Job drawing, mm, ordinate dimensions from the low corner. One solid piece. A direction names the side the tool comes from. Coordinates: 2 decimals unless noted, no trailing zeros. Write each loop counter-clockwise with the first axis right and the second up, starting at its lowest first coordinate (ties: lowest second). Pieces come first, ordered by that corner, then holes. Notation, with made-up numbers: (83, -38) - (124, -38) arc R17 cw to (124, -12) - close; hole circle Ø3 at (-20, 26.5). An arc over 180 degrees is marked (long way). Put each result on its own line as item: value. Start each with the question number.
1. Drop flat-ended pins along their axis: P1, Ø12, axis at y = 4, z = 52, coming from the +X side; P2, Ø9, axis at x = 21, y = 20.5, coming from the +Z side; P3, Ø3, axis at y = 8.5, z = 58.5, coming from the +X side. Give the stop position or say it passes through.
2. Saw through at B-B, the plane z = 33. Write the cut outline in (x, y), plus the area to 3 significant figures.
3. Saw through at C-C, the plane x = 54.5. Write the cut outline in (y, z), plus the area to 3 significant figures.
4. Saw through at A-A, the plane y = 9. Write the cut outline in (x, z).
5. Saw through at D-D, the plane z = 63. Write the cut outline in (x, y), plus the area to 3 significant figures.
6. Which spindle directions (+Z, -Z, +X, -X, +Y, -Y) get a long thin tool onto all of the face, cutting with end or side? Do the marked faces 1 and 2. Say none if no direction does.
7. Drill centre lines: L1, parallel to Z at x = 29, y = 10.25; L2, parallel to X at y = 16.5, z = 66; L3, parallel to X at y = 15.5, z = 35. Where is each one in solid material? Low to high. Write a range as from..to.
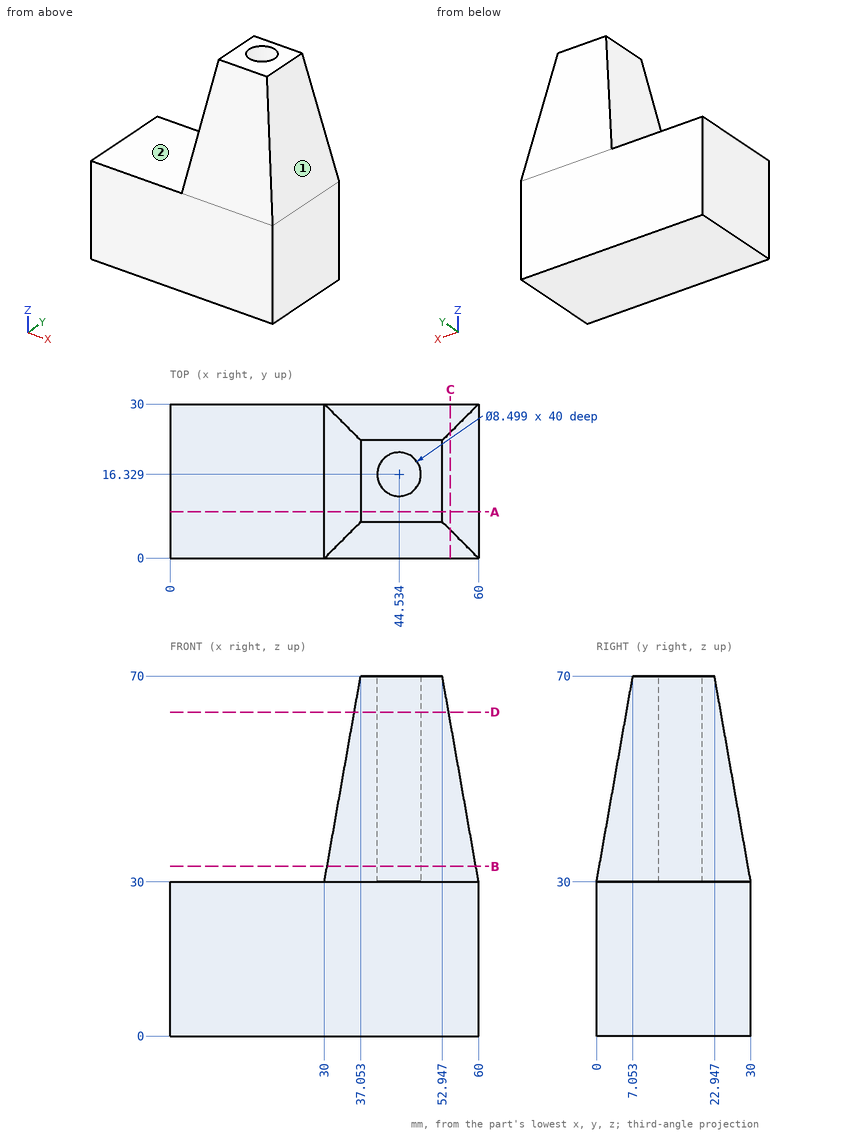
Final values:
1. P1: stops at x = 57.18
1. P2: stops at z = 30
1. P3: stops at x = 55.24
2. outline: (30.53, 0.53) - (59.47, 0.53) - (59.47, 29.47) - (30.53, 29.47) - close; hole circle Ø8.5 at (44.53, 16.33)
2. area: 781 mm²
3. outline: (0, 0) - (30, 0) - (30, 30) - (24.5, 61.19) - (5.5, 61.19) - (0, 30) - close
3. area: 1,660 mm²
4. outline: (0, 0) - (60, 0) - (60, 30) - (52.95, 70) - (37.05, 70) - (30, 30) - (0, 30) - close
5. outline: (35.82, 5.82) - (54.18, 5.82) - (54.18, 24.18) - (35.82, 24.18) - close; hole circle Ø8.5 at (44.53, 16.33)
5. area: 280 mm²
6. face 1: +Z, +X, +Y, -Y
6. face 2: +Z, -X, +Y, -Y
7. L1: z = 0..30
7. L2: x = 36.35..40.29, 48.78..53.65
7. L3: x = 30.88..40.37, 48.7..59.12
